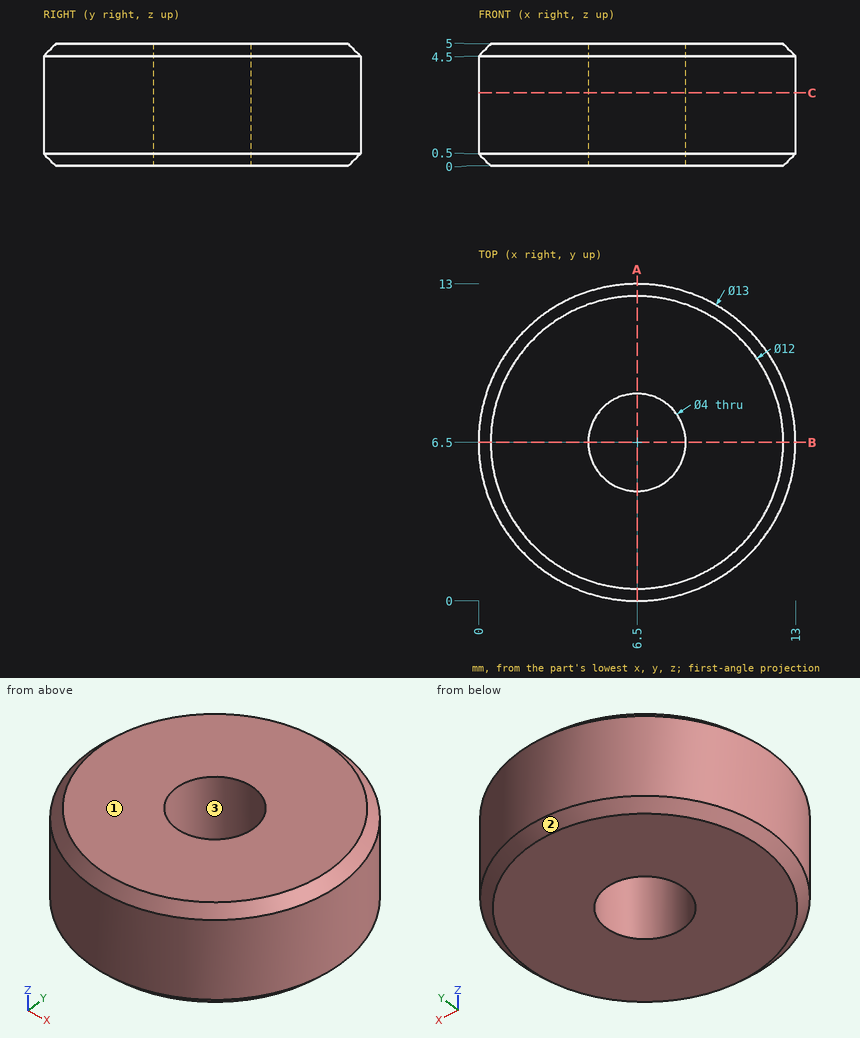
Verification items for this drawing (mm, ordinates from the low corner). Round coordinates to 2 decimals unless told otherwise and drop trailing zeros. Order: outer loops, then holes, each group sorted by start corner. A loop starts at its lowest first (then second) coordinate and runs counter-clockwise, first axis right, second up. Notation, with made-up numbers: M 7.5,76.5 L 45.5,76.5 A11 cw 45.5,97.5 Z; hole C 45,32.5 d5. An arc over 180 degrees is marked long. Answer in a Markdown table with one row per item. Add a question column.
Item 1: Draft check along Y on the marked faces 1, 2 and 3. Enter one of: released by +Y, released by -Y, zero draft, split by the parting line, or undercut.
Item 2: Sectioned sample at A-A, the plane x = 6.5. Enter the section's corners in (y, z).
Item 3: Sectioned sample at C-C, the plane z = 3. Enter the section's corners in (x, y).
Item 4: Material ranges on L1, parallel to Y at x = 6.5, z = 2.4; L2, parallel to X at y = 6.75, z = 4.3; L3, parallel to X at y = 4, z = 1.45, recorded low to high. Write a range as [from, to].
Item 5: Depth check by flat-ended pin: pin 1 Ø2 at (y, z) = (9.5, 4) entering from +X; pin 2 Ø6 at (x, y) = (7, 7) entering from -Z; pin 3 Ø3 at (y, z) = (4, 4) entering from +X. Enter the tip coordinate at first touch or a pass-through.
Filled in:
| question | item | result |
|---|---|---|
| 1 | face 1 | zero draft |
| 1 | face 2 | split by the parting line |
| 1 | face 3 | undercut |
| 2 | outline | M 0,0.5 L 0.5,0 L 4.5,0 L 4.5,5 L 0.5,5 L 0,4.5 Z; M 8.5,0 L 12.5,0 L 13,0.5 L 13,4.5 L 12.5,5 L 8.5,5 Z |
| 3 | outline | C 6.5,6.5 d13; hole C 6.5,6.5 d4 |
| 4 | L1 | y = [0, 4.5], [8.5, 13] |
| 4 | L2 | x = [0, 4.52], [8.48, 13] |
| 4 | L3 | x = [0.5, 12.5] |
| 5 | pin 1 | stops at x = 12.68 |
| 5 | pin 2 | stops at z = 0 |
| 5 | pin 3 | stops at x = 12.92 |
